Design review of the part built by this model. Coordinates are the model's own, in mm. A direction names the side the tool comes from. Give positions to 0.01 mm unless a question says otherwise; leave off trailing zeros. Write each loop counter-clockwise with the first axis right and the second up, starting at its lowest first coordinate (ties: lowest second). Pieces come first, ordered by that corner, then holes. Notation, with made-up numbers: (-34.5, 23.5) - (23.5, 23.5) arc R15 cw to (23.5, 41.5) - close; hole circle Ø4 at (86, -25). An arc over 180 degrees is marked (long way). Use a Markdown table: item, result. Add a question column.
```python
from build123d import *

# Parameters (mm, degrees)
SKETCH1_W           = 20
SKETCH1_H           = 50
BOSS_EXTRUDE1_DEPTH = 70
SKETCH2_R           = 2
SKETCH2_R_2         = 11.5
CUT_EXTRUDE2_DEPTH  = 60
SKETCH4_W           = 38
SKETCH4_H           = 15
CUT_EXTRUDE3_DEPTH  = 60
SKETCH8_R           = 2
CUT_EXTRUDE5_DEPTH  = 15
SKETCH9_W           = 42
SKETCH9_H           = 42
CUT_EXTRUDE6_DEPTH  = 6
SKETCH10_R          = 2
CUT_EXTRUDE7_DEPTH  = 7
CUT_EXTRUDE8_DEPTH  = 30
SKETCH12_W          = 20
SKETCH12_H          = 5
BOSS_EXTRUDE2_DEPTH = 10
BOSS_EXTRUDE3_DEPTH = 20
SKETCH15_R          = 2
CUT_EXTRUDE9_DEPTH  = 10


with BuildPart() as part:
    # Sketch1 → Boss-Extrude1 (new body)
    with BuildSketch(Plane(origin=(0, 0, 0), x_dir=(1, 0, 0), z_dir=(0, 1, 0))):
        with Locations((-10, -25)):
            Rectangle(SKETCH1_W, SKETCH1_H)
    extrude(amount=BOSS_EXTRUDE1_DEPTH)

    # Sketch2 → Cut-Extrude2 (cut)
    with BuildSketch(Plane(origin=(0, 0, 0), x_dir=(0, 0, -1), z_dir=(1, 0, 0))):
        with Locations((-9.5, 58)):
            Circle(SKETCH2_R)
        with Locations((-25, 42.5)):
            Circle(SKETCH2_R_2)
        with Locations((-9.5, 27)):
            Circle(SKETCH2_R)
        with Locations((-40.5, 27)):
            Circle(SKETCH2_R)
        with Locations((-40.5, 58)):
            Circle(SKETCH2_R)
    extrude(amount=-CUT_EXTRUDE2_DEPTH, mode=Mode.SUBTRACT)

    # Sketch4 → Cut-Extrude3 (cut)
    with BuildSketch(Plane(origin=(0, 0, 0), x_dir=(0, 0, -1), z_dir=(1, 0, 0))):
        with Locations((-31, 7.5)):
            Rectangle(SKETCH4_W, SKETCH4_H)
    extrude(amount=-CUT_EXTRUDE3_DEPTH, mode=Mode.SUBTRACT)

    # Sketch8 → Cut-Extrude5 (cut)
    with BuildSketch(Plane(origin=(0, 0, 0), x_dir=(-1, 0, 0), z_dir=(0, 0, -1))):
        with Locations((15, 6)):
            Circle(SKETCH8_R)
    extrude(amount=-CUT_EXTRUDE5_DEPTH, mode=Mode.SUBTRACT)

    # Sketch9 → Cut-Extrude6 (cut)
    with BuildSketch(Plane(origin=(0, 0, 0), x_dir=(0, 0, -1), z_dir=(1, 0, 0))):
        with Locations((-25, 42.5)):
            Rectangle(SKETCH9_W, SKETCH9_H)
    extrude(amount=-CUT_EXTRUDE6_DEPTH, mode=Mode.SUBTRACT)

    # Sketch10 → Cut-Extrude7 (cut)
    with BuildSketch(Plane(origin=(0, 0, 0), x_dir=(-1, 0, 0), z_dir=(0, 0, -1))):
        with Locations((5, 6)):
            Circle(SKETCH10_R)
    extrude(amount=-CUT_EXTRUDE7_DEPTH, mode=Mode.SUBTRACT)

    # Sketch11 → Cut-Extrude8 (cut)
    with BuildSketch(Plane(origin=(0, 0, 0), x_dir=(0, 0, -1), z_dir=(1, 0, 0))):
        Polygon((-6, 0), (0, 0), (0, 15), align=None)
    extrude(amount=-CUT_EXTRUDE8_DEPTH, mode=Mode.SUBTRACT)

    # Sketch12 → Boss-Extrude2 (add)
    with BuildSketch(Plane.XY.offset(50)):
        with Locations((-10, 17.5)):
            Rectangle(SKETCH12_W, SKETCH12_H)
    extrude(amount=BOSS_EXTRUDE2_DEPTH)

    # Sketch14 → Boss-Extrude3 (add)
    with BuildSketch(Plane(origin=(0, 0, 0), x_dir=(0, 0, -1), z_dir=(1, 0, 0))):
        Polygon((-50, 20), (-60, 20), (-50, 25), align=None)
    extrude(amount=-BOSS_EXTRUDE3_DEPTH)

    # Sketch15 → Cut-Extrude9 (cut)
    with BuildSketch(Plane(origin=(0, 15, 0), x_dir=(-1, 0, 0), z_dir=(0, -1, 0))):
        with Locations(Location((5, -55, 0), (0, 0, 90))):
            Circle(SKETCH15_R)
        with Locations(Location((15, -55, 0), (0, 0, 90))):
            Circle(SKETCH15_R)
    extrude(amount=-CUT_EXTRUDE9_DEPTH, mode=Mode.SUBTRACT)


solid = part.part
```
(1) Mouldability with a two-part tool opening along Y and no side actions: class faces 1 (the face through (-9.86, 22.465, 55.07)), 2 (the face through (-10, 47, 50)), 3 (the face through (-3, 63.5, 25)) as +Y half, -Y half, draft (parallel to the pull), parting line (faces both ways), or undercut.
(2) Add section D-D (y = 6). State the section outline as (x, z) points.
(3) Insertion check: pin 1 (12 mm diameter, centred on x = -4.5, y = 50.5, fed in from +Z); pin 2 (6.5 mm diameter, centred on y = 27, z = 9.5, fed in from +X); pin 3 (4.5 mm diameter, centred on x = -5, z = 55, fed in from -Y). Each pin has a flat end and moves straight along its axis. Give the tip position at first contact, or say it passes through.
(4) Add section B-B (x = -15). State the section outline as (y, z) points, and give its area (3 significant figures).
(5) For line 1 along X through (y, z) = (6, 4.9); line 2 along Y through (x, z) = (-10.25, 9.5); line 3 along Y through (x, z) = (-1.25, 16), list the stretches that pass through material, from the lowest coordinate up.
(6) Add section C-C (z = 40.5). State the section outline as (x, y) points, and give its area (3 significant figures).
(7) Tool access review of faces 4 (the face through (-3, 21.5, 25)), 5 (the face through (-15, 8, 7)), 6 (the face through (-12.902, 25.048, 40.934)), 7 (the face through (-10, 7, 12)), 8 (the face through (-5, 6, 7)): name each direction out of +Z, -Z, +X, -X, +Y, -Y from which nothing blocks a thin tool from reaching the whole face with its end or side.
(8) Add section A-A (x = -5). State the section outline as (y, z) points.
Answers follow:
| question | item | result |
|---|---|---|
| 1 | face 1 | +Y half |
| 1 | face 2 | draft |
| 1 | face 3 | undercut |
| 2 | outline | (-20, 3.6) - (-17, 3.6) - (-17, 12) - (-20, 12) - close; (-13, 3.6) - (-7, 3.6) - (-7, 7) - (-3, 7) - (-3, 3.6) - (0, 3.6) - (0, 12) - (-13, 12) - close |
| 3 | pin 1 | z = 50 |
| 3 | pin 2 | x = -6 |
| 3 | pin 3 | y = 15 |
| 4 | outline | (0, 6) - (4, 4.4) - (4, 12) - (0, 12) - close; (8, 2.8) - (15, 0) - (70, 0) - (70, 50) - (25, 50) - (23.5, 53) - (15, 53) - (15, 12) - (8, 12) - close; (15, 57) - (21.5, 57) - (20, 60) - (15, 60) - close; hole circle Ø4 at (27, 9.5); hole circle Ø4 at (27, 40.5); hole circle Ø23 at (42.5, 25); hole circle Ø4 at (58, 9.5); hole circle Ø4 at (58, 40.5) |
| 4 | area | 2,430 mm^2 |
| 5 | line 1 | -20 to -17, -13 to -7, -3 to 0 |
| 5 | line 2 | 0 to 25, 29 to 56, 60 to 70 |
| 5 | line 3 | 15 to 21.5, 63.5 to 70 |
| 6 | outline | (-20, 15) - (0, 15) - (0, 21.5) - (-6, 21.5) - (-6, 25) - (-20, 25) - close; (-20, 29) - (-6, 29) - (-6, 56) - (-20, 56) - close; (-20, 60) - (-6, 60) - (-6, 63.5) - (0, 63.5) - (0, 70) - (-20, 70) - close |
| 6 | area | 736 mm^2 |
| 7 | face 4 | +X |
| 7 | face 5 | +Z, -Z |
| 7 | face 6 | +X, -X |
| 7 | face 7 | +Z, +X, -X, -Y |
| 7 | face 8 | -Z |
| 8 | outline | (0, 6) - (4, 4.4) - (4, 7) - (8, 7) - (8, 2.8) - (15, 0) - (70, 0) - (70, 50) - (25, 50) - (23.5, 53) - (15, 53) - (15, 12) - (0, 12) - close; (15, 57) - (21.5, 57) - (20, 60) - (15, 60) - close; hole (21.5, 4) - (63.5, 4) - (63.5, 46) - (21.5, 46) - close |
